```python
from build123d import *

# Parameters (mm, degrees)
BOSS_EXTRUDE1_DEPTH = 2
SKETCH3_R           = 1.25
CUT_EXTRUDE1_DEPTH  = 188.552659272


with BuildPart() as part:
    # Sketch2 → Boss-Extrude1 (new body)
    with BuildSketch(Plane.XY):
        with BuildLine():
            Line((-79.195959493, 62.225396744), (-62.225396744, 79.195959493))
            ThreePointArc((-62.225396744, 79.195959493), (-44.806778225, 80.702789346), (-30, 90))
            Line((-30, 90), (30, 90))
            ThreePointArc((30, 90), (44.806778225, 80.702789346), (62.225396744, 79.195959493))
            Line((62.225396744, 79.195959493), (79.195959493, 62.225396744))
            ThreePointArc((79.195959493, 62.225396744), (58.781303002, 0), (79.195959493, -62.225396744))
            Line((79.195959493, -62.225396744), (62.225396744, -79.195959493))
            ThreePointArc((62.225396744, -79.195959493), (43.875108319, -77.923881554), (30, -90))
            Line((30, -90), (30, -155))
            ThreePointArc((30, -155), (25.606601718, -165.606601718), (15, -170))
            Line((15, -170), (-15, -170))
            ThreePointArc((-15, -170), (-25.606601718, -165.606601718), (-30, -155))
            Line((-30, -155), (-30, -90))
            ThreePointArc((-30, -90), (-43.875108319, -77.923881554), (-62.225396744, -79.195959493))
            Line((-62.225396744, -79.195959493), (-79.195959493, -62.225396744))
            ThreePointArc((-79.195959493, -62.225396744), (-58.781303002, 0), (-79.195959493, 62.225396744))
        make_face()
    extrude(amount=BOSS_EXTRUDE1_DEPTH)

    # Sketch3 → Cut-Extrude1 (cut, through all)
    with BuildSketch(Plane.XY.offset(2)):
        with Locations((-73.892658634, 61.871843354)):
            Circle(SKETCH3_R)
        with Locations((-59.75052301, 47.72970773)):
            Circle(SKETCH3_R)
        with Locations(Location((-61.871843354, 73.892658634, 0), (0, 0, 180))):
            Circle(SKETCH3_R)
        with Locations(Location((-47.72970773, 59.75052301, 0), (0, 0, 180))):
            Circle(SKETCH3_R)
        with Locations(Location((59.75052301, 47.72970773, 0), (0, 0, 180))):
            Circle(SKETCH3_R)
        with Locations(Location((73.892658634, 61.871843354, 0), (0, 0, 180))):
            Circle(SKETCH3_R)
        with Locations((61.871843354, 73.892658634)):
            Circle(SKETCH3_R)
        with Locations((47.72970773, 59.75052301)):
            Circle(SKETCH3_R)
        with Locations(Location((-59.75052301, -47.72970773, 0), (0, 0, 180))):
            Circle(SKETCH3_R)
        with Locations((-47.72970773, -59.75052301)):
            Circle(SKETCH3_R)
        with Locations((-61.871843354, -73.892658634)):
            Circle(SKETCH3_R)
        with Locations(Location((-73.892658634, -61.871843354, 0), (0, 0, 180))):
            Circle(SKETCH3_R)
        with Locations((59.75052301, -47.72970773)):
            Circle(SKETCH3_R)
        with Locations((73.892658634, -61.871843354)):
            Circle(SKETCH3_R)
        with Locations(Location((61.871843354, -73.892658634, 0), (0, 0, 180))):
            Circle(SKETCH3_R)
        with Locations(Location((47.72970773, -59.75052301, 0), (0, 0, 180))):
            Circle(SKETCH3_R)
    extrude(amount=-CUT_EXTRUDE1_DEPTH, mode=Mode.SUBTRACT)


solid = part.part
```
Work out the finished part from the listing and answer in its coordinate system (mm). Round coordinates to 2 decimals unless told otherwise and drop trailing zeros. Write each loop counter-clockwise with the first axis right and the second up, starting at its lowest first coordinate (ties: lowest second). Pieces come first, ordered by that corner, then holes.
1) A cutting plane is placed at A-A on z = 0.7. Give the number of separate pieces and of enclosed holes in the cut face, and give its area (3 significant figures).
2) Consider probe 1 along X at (y, z) = (1.5, 1.6); probe 2 along Y at (x, z) = (66, 1.6); probe 3 along Y at (x, z) = (51, 0.55). Determine where each line is inside the solid, lowest interval first.
3) A cutting plane is placed at C-C on x = -37.5. Determine the outline of the cut face in (y, z).
4) A cutting plane is placed at B-B on y = -123. Determine the outline of the cut face in (x, z).
5) Flat-ended cylindrical pins translate along their axes: P1, Ø2, axis at x = -61.87, y = -73.89, coming from the +Z side; P2, Ø1, axis at y = -120.5, z = 1, coming from the +X side. Find the tip coordinate at first contact, or state that the pin passes through.
6) Determine the mould class of faces 1 (the face through (-43.625, -78.009, 0.986)), 2 (the face through (1, -9, 2)), 3 (the face through (-70.83, 70.59, 0.99)), 4 (the face through (25.72, -165.49, 0.99)) for opening direction X: pulls with the +X half, pulls with the -X half, needs draft (parallel to the pull), parting line crosses it, or undercut.
Entries:
1. separate pieces: 1
1. enclosed holes: 16
1. area: 27,200 mm2
2. probe 1: x = -58.79 to 58.79
2. probe 2: y = -75.42 to -38.27, 38.27 to 75.42
2. probe 3: y = -76.68 to 79.2
3. outline: (-81.19, 0) - (84.07, 0) - (84.07, 2) - (-81.19, 2) - close
4. outline: (-30, 0) - (30, 0) - (30, 2) - (-30, 2) - close
5. P1: passes through
5. P2: stops at x = 30
6. face 1: undercut
6. face 2: needs draft
6. face 3: pulls with the -X half
6. face 4: pulls with the +X half
